from build123d import *

# Parameters (mm, degrees)
BOSS_EXTRUDE1_DEPTH  = 2.8
BOSS_EXTRUDE5_DEPTH  = 2.8
BOSS_EXTRUDE2_DEPTH  = 2.8
BOSS_EXTRUDE3_DEPTH  = 2.8
BOSS_EXTRUDE4_DEPTH  = 2.8
BOSS_EXTRUDE6_DEPTH  = 11.2
BOSS_EXTRUDE7_START  = -2.8
BOSS_EXTRUDE7_DEPTH  = 2.8
BOSS_EXTRUDE8_START  = 11.2
BOSS_EXTRUDE8_DEPTH  = 11.2
BOSS_EXTRUDE9_START  = 8.4
BOSS_EXTRUDE9_DEPTH  = 8.4
BOSS_EXTRUDE10_START = 5.6
BOSS_EXTRUDE10_DEPTH = 5.6
BOSS_EXTRUDE11_START = 2.8
BOSS_EXTRUDE11_DEPTH = 2.8


with BuildPart() as part:
    # Sketch1 → Boss-Extrude1 (new body)
    with BuildSketch(Plane.XY):
        with BuildLine():
            Line((-31.75, 18.9), (31.75, 18.9))
            ThreePointArc((31.75, 18.9), (50.65, 0), (31.75, -18.9))
            Line((31.75, -18.9), (-31.75, -18.9))
            ThreePointArc((-31.75, -18.9), (-50.65, 0), (-31.75, 18.9))
        make_face()
    extrude(amount=BOSS_EXTRUDE1_DEPTH)

    # Sketch5 → Boss-Extrude5 (add)
    with BuildSketch(Plane(origin=(0, 0, 0), x_dir=(-1, 0, 0), z_dir=(0, 0, -1))):
        with BuildLine():
            Line((-46.65, -13.7), (-46.65, 13.7))
            ThreePointArc((-46.65, 13.7), (-37.937921505, 29.619053219), (-19.833465037, 30.862123242))
            Line((-19.833465037, 30.862123242), (9.866534963, 17.162123242))
            ThreePointArc((9.866534963, 17.162123242), (20.85, 0), (9.866534963, -17.162123242))
            Line((9.866534963, -17.162123242), (-19.833465037, -30.862123242))
            ThreePointArc((-19.833465037, -30.862123242), (-37.937921505, -29.619053219), (-46.65, -13.7))
        make_face()
    extrude(amount=BOSS_EXTRUDE5_DEPTH)

    # Sketch2 → Boss-Extrude2 (add)
    with BuildSketch(Plane.XY.offset(2.8)):
        with BuildLine():
            Line((-45.25, 18.9), (45.25, 18.9))
            ThreePointArc((45.25, 18.9), (64.15, 0), (45.25, -18.9))
            Line((45.25, -18.9), (-45.25, -18.9))
            ThreePointArc((-45.25, -18.9), (-64.15, 0), (-45.25, 18.9))
        make_face()
    extrude(amount=BOSS_EXTRUDE2_DEPTH)

    # Sketch3 → Boss-Extrude3 (add)
    with BuildSketch(Plane.XY.offset(5.6)):
        with BuildLine():
            Line((-58.75, 18.9), (58.75, 18.9))
            ThreePointArc((58.75, 18.9), (77.65, 0), (58.75, -18.9))
            Line((58.75, -18.9), (-58.75, -18.9))
            ThreePointArc((-58.75, -18.9), (-77.65, 0), (-58.75, 18.9))
        make_face()
    extrude(amount=BOSS_EXTRUDE3_DEPTH)

    # Sketch4 → Boss-Extrude4 (add)
    with BuildSketch(Plane.XY.offset(8.4)):
        with BuildLine():
            Line((-72.75, 18.9), (72.75, 18.9))
            ThreePointArc((72.75, 18.9), (91.65, 0), (72.75, -18.9))
            Line((72.75, -18.9), (-72.75, -18.9))
            ThreePointArc((-72.75, -18.9), (-91.65, 0), (-72.75, 18.9))
        make_face()
    extrude(amount=BOSS_EXTRUDE4_DEPTH)

    # Sketch7 → Boss-Extrude6 (add)
    with BuildSketch(Plane.XY):
        with BuildLine():
            Line((31.75, -18.9), (-6.099021116, -18.9))
            Line((-6.099021116, -18.9), (19.833465037, -30.862123242))
            ThreePointArc((19.833465037, -30.862123242), (37.937921505, -29.619053219), (46.65, -13.7))
            Line((46.65, -13.7), (46.65, -11.627553483))
            ThreePointArc((46.65, -11.627553483), (40.040031338, -16.984857386), (31.75, -18.9))
        make_face()
        with BuildLine():
            Line((46.65, 11.627553483), (46.65, 13.7))
            ThreePointArc((46.65, 13.7), (37.937921505, 29.619053219), (19.833465037, 30.862123242))
            Line((19.833465037, 30.862123242), (-6.099021116, 18.9))
            Line((-6.099021116, 18.9), (31.75, 18.9))
            ThreePointArc((31.75, 18.9), (40.040031338, 16.984857386), (46.65, 11.627553483))
        make_face()
    extrude(amount=BOSS_EXTRUDE6_DEPTH)

    # Sketch10 → Boss-Extrude7 (add)
    with BuildSketch(Plane(origin=(0, 0, -2.8), x_dir=(-1, 0, 0), z_dir=(0, 0, -1)).offset(BOSS_EXTRUDE7_START)):
        with BuildLine():
            ThreePointArc((18.009763314, -9.964637591), (28.85, 0), (18.009763314, 9.964637591))
            ThreePointArc((18.009763314, 9.964637591), (20.85, 0), (18.009763314, -9.964637591))
        make_face()
    extrude(amount=BOSS_EXTRUDE7_DEPTH)

    # Sketch11 → Boss-Extrude8 (add)
    with BuildSketch(Plane(origin=(0, 0, 8.4), x_dir=(-1, 0, 0), z_dir=(0, 0, -1)).offset(BOSS_EXTRUDE8_START)):
        with BuildLine():
            Line((-72.75, -18.7), (-72.75, -18.9))
            ThreePointArc((-72.75, -18.9), (-91.65, 0), (-72.75, 18.9))
            Line((-72.75, 18.9), (-72.75, 18.7))
            ThreePointArc((-72.75, 18.7), (-91.45, 0), (-72.75, -18.7))
        make_face()
        with BuildLine():
            Line((72.75, -18.7), (72.75, -18.9))
            ThreePointArc((72.75, -18.9), (91.65, 0), (72.75, 18.9))
            Line((72.75, 18.9), (72.75, 18.7))
            ThreePointArc((72.75, 18.7), (91.45, 0), (72.75, -18.7))
        make_face()
    extrude(amount=-BOSS_EXTRUDE8_DEPTH)

    # Sketch12 → Boss-Extrude9 (add)
    with BuildSketch(Plane(origin=(0, 0, 5.6), x_dir=(-1, 0, 0), z_dir=(0, 0, -1)).offset(BOSS_EXTRUDE9_START)):
        with BuildLine():
            Line((-58.75, 18.9), (-58.75, 18.7))
            ThreePointArc((-58.75, 18.7), (-77.45, 0), (-58.75, -18.7))
            Line((-58.75, -18.7), (-58.75, -18.9))
            ThreePointArc((-58.75, -18.9), (-77.65, 0), (-58.75, 18.9))
        make_face()
        with BuildLine():
            Line((58.75, 18.9), (58.75, 18.7))
            ThreePointArc((58.75, 18.7), (77.45, 0), (58.75, -18.7))
            Line((58.75, -18.7), (58.75, -18.9))
            ThreePointArc((58.75, -18.9), (77.65, 0), (58.75, 18.9))
        make_face()
    extrude(amount=-BOSS_EXTRUDE9_DEPTH)

    # Sketch13 → Boss-Extrude10 (add)
    with BuildSketch(Plane(origin=(0, 0, 2.8), x_dir=(-1, 0, 0), z_dir=(0, 0, -1)).offset(BOSS_EXTRUDE10_START)):
        with BuildLine():
            Line((-45.924016822, 18.887977693), (-45.916884369, 18.688104913))
            ThreePointArc((-45.916884369, 18.688104913), (-63.95, 0), (-45.916884369, -18.688104913))
            Line((-45.916884369, -18.688104913), (-45.924016822, -18.887977693))
            ThreePointArc((-45.924016822, -18.887977693), (-64.15, 0), (-45.924016822, 18.887977693))
        make_face()
        with BuildLine():
            Line((45.25, 18.9), (45.25, 18.7))
            ThreePointArc((45.25, 18.7), (63.95, 0), (45.25, -18.7))
            Line((45.25, -18.7), (45.25, -18.9))
            ThreePointArc((45.25, -18.9), (64.15, 0), (45.25, 18.9))
        make_face()
    extrude(amount=-BOSS_EXTRUDE10_DEPTH)

    # Sketch14 → Boss-Extrude11 (add)
    with BuildSketch(Plane(origin=(0, 0, 0), x_dir=(-1, 0, 0), z_dir=(0, 0, -1)).offset(BOSS_EXTRUDE11_START)):
        with BuildLine():
            Line((-46.65, -11.627553483), (-46.492328042, -11.504510589))
            ThreePointArc((-46.492328042, -11.504510589), (-50.45, 0), (-46.492328042, 11.504510589))
            Line((-46.492328042, 11.504510589), (-46.65, 11.627553483))
            ThreePointArc((-46.65, 11.627553483), (-50.65, 0), (-46.65, -11.627553483))
        make_face()
        with BuildLine():
            Line((31.75, 18.9), (31.75, 18.7))
            ThreePointArc((31.75, 18.7), (50.45, 0), (31.75, -18.7))
            Line((31.75, -18.7), (31.75, -18.9))
            ThreePointArc((31.75, -18.9), (50.65, 0), (31.75, 18.9))
        make_face()
    extrude(amount=-BOSS_EXTRUDE11_DEPTH)


solid = part.part
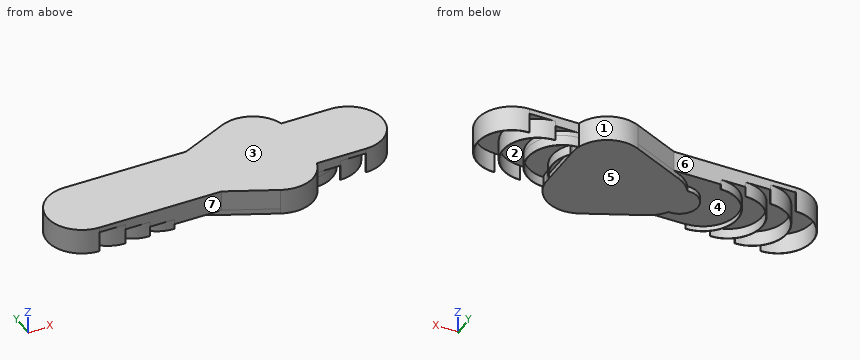
CAD build for the part. Positions are in the model's coordinates, mm. Face numbers are marked on the shaded views. A direction names the side the tool comes from. Give positions to 0.01 mm unless a question says otherwise; leave off trailing zeros. Write each loop counter-clockwise with the first axis right and the second up, starting at its lowest first coordinate (ties: lowest second). Pieces come first, ordered by that corner, then holes. Notation, with made-up numbers: M 43.25,34.25 L 74.25,34.25 A6 ccw 74.25,45.25 Z; hole C -36.75,16.25 d6. An arc over 180 degrees is marked long. Put each result on its own line as item: value. Start each with the question number.
(1) Band-saw the part on C-C, the plane y = 22. Write the cut outline in (x, z).
(2) Band-saw the part on B-B, the plane y = 29. Write the cut outline in (x, z).
(3) Probe L1, parallel to X at y = 8.5, z = 7; L2, parallel to X at y = 15.5, z = 7.5; L3, parallel to Z at x = -37, y = -2.5. List the from-to ranges inside material, lowest first.
(4) Mould opens along X. For the marked faces 1, 2 and 3 say: +X half, -X half, draft (parallel to the pull), parting line (faces both ways), or undercut.
(5) Flat gauge pins, fed straight in: pin 1 Ø1 at (x, z) = (6, 5.5) entering from +Y; pin 2 Ø6 at (y, z) = (11, -1) entering from -X; pin 3 Ø8 at (x, z) = (17.5, 5.5) entering from -Y; pin 4 Ø1.5 at (x, y) = (4, 25) entering from -Z. Where does each tip first touch, or does it go through?
(6) Which spindle directions (+Z, -Z, +X, -X, +Y, -Y) get a long thin tool onto all of the face, cutting with end or side? Do the marked faces 4, 5, 6 and 7. Say none if no direction does.
(7) Band-saw the part on A-A, the plane x = 67. Write the cut outline in (y, z), and give its area (3 significant figures).
Response values:
1. outline: M 0.62,-2.8 L 44.73,-2.8 L 44.73,11.2 L 0.62,11.2 Z
2. outline: M 15.8,-2.8 L 38.85,-2.8 L 38.85,11.2 L 15.8,11.2 Z
3. L1: x = -89.63 to -89.41, -75.63 to 75.63, 89.41 to 89.63
3. L2: x = -83.56 to -83.21, -69.56 to 69.56, 83.21 to 83.56
3. L3: z = 0 to 11.2
4. face 1: parting line
4. face 2: undercut
4. face 3: draft
5. pin 1: stops at y = 24.71
5. pin 2: stops at x = -89.87
5. pin 3: stops at y = -31.54
5. pin 4: passes through
6. face 4: -Z
6. face 5: -Z, +X, -X, +Y, -Y
6. face 6: +Z, -Z, -X, +Y
6. face 7: +Z, -Z, -X, -Y
7. outline: M -18.9,8.4 L -17,8.4 L -17,-2.8 L -16.78,-2.8 L -16.78,5.6 L 16.78,5.6 L 16.78,-2.8 L 17,-2.8 L 17,8.4 L 18.9,8.4 L 18.9,11.2 L -18.9,11.2 Z
7. area: 205 mm2
